Verification items for the finished model (mm, model axes). Face numbers are marked on the shaded views. A direction names the side the tool comes from. Round coordinates to 2 decimals unless told otherwise and drop trailing zeros. Write each loop counter-clockwise with the first axis right and the second up, starting at its lowest first coordinate (ties: lowest second). Pieces come first, ordered by that corner, then holes. Notation, with made-up numbers: (-37, 18) - (21, 18) arc R29 cw to (21, 53) - close; hole circle Ø11 at (-33.5, -27). An arc over 180 degrees is marked (long way). Answer as a JSON object with one key per item and string values.
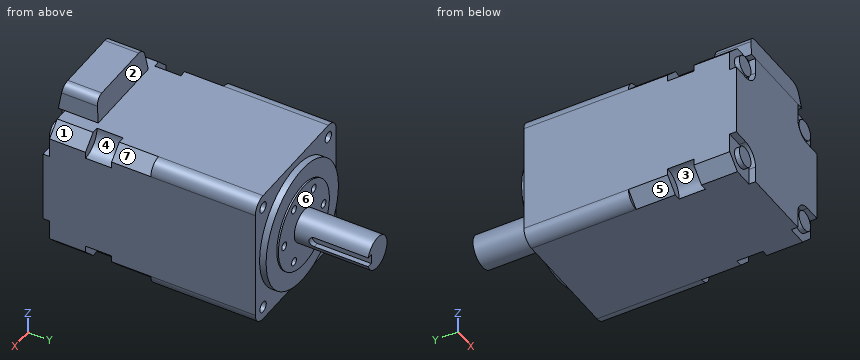
```python
from build123d import *

# Parameters (mm, degrees)
EXTRUDE_1_DEPTH          = 65
CUT_EXTRUDE_1_DEPTH      = 33
CUT_EXTRUDE_START        = -13
CUT_EXTRUDE_2_DEPTH      = 8
CUT_EXTRUDE_3_DEPTH      = 2
SKETCH_5_R               = 3
EXTRUDE_2_DEPTH          = 1.5
SKETCH_6_W               = 26
SKETCH_6_H               = 12.2
EXTRUDE_3_DEPTH          = 7.5
CUT_EXTRUDE_4_REACH      = 80.697
CUT_EXTRUDE_5_REACH      = 76.015
FILLET_2_R               = 2.8
SKETCH_10_R              = 18.8
EXTRUDE_4_DEPTH          = 2
SKETCH_11_R              = 13.25
EXTRUDE_5_DEPTH          = 0.5
SKETCH_12_R              = 5
EXTRUDE_6_DEPTH          = 22.5
CUT_EXTRUDE_6_REACH      = 101.912
CUT_EXTRUDE_6_END_RADIUS = 5
CUT_EXTRUDE_START_2      = 3.2
HOLE_WIZARD_M3_2_D       = 2.5
HOLE_WIZARD_M3_2_DEPTH   = 6.5
HOLE_WIZARD_M3_2_TIP     = 0.751075774
HOLE_WIZARD_M4_1_D       = 3.3
HOLE_WIZARD_M4_1_DEPTH   = 10
HOLE_WIZARD_M4_1_TIP     = 0.991420021


with BuildPart() as part:
    # 草图1 → 凸台-拉伸1 (new body)
    with BuildSketch(Plane(origin=(0, 0, 0), x_dir=(1, 0, 0), z_dir=(0, 1, 0))):
        with BuildLine():
            Line((17, -21), (-17, -21))
            ThreePointArc((-17, -21), (-19.828427125, -19.828427125), (-21, -17))
            Line((-21, -17), (-21, 17))
            ThreePointArc((-21, 17), (-19.828427125, 19.828427125), (-17, 21))
            Line((-17, 21), (17, 21))
            ThreePointArc((17, 21), (19.828427125, 19.828427125), (21, 17))
            Line((21, 17), (21, -17))
            ThreePointArc((21, -17), (19.828427125, -19.828427125), (17, -21))
        make_face()
    extrude(amount=EXTRUDE_1_DEPTH)

    # 草图2 → 切除-拉伸1 (cut)
    with BuildSketch(Plane.XZ):
        with BuildLine():
            Line((-17, 21), (-21, 17))
            ThreePointArc((-21, 17), (-19.828427125, 19.828427125), (-17, 21))
        make_face()
        with BuildLine():
            Line((17, 21), (21, 17))
            ThreePointArc((21, 17), (19.828427125, 19.828427125), (17, 21))
        make_face()
        with BuildLine():
            Line((-21, -17), (-17, -21))
            ThreePointArc((-17, -21), (-19.828427125, -19.828427125), (-21, -17))
        make_face()
        with BuildLine():
            Line((21, -17), (17, -21))
            ThreePointArc((17, -21), (19.828427125, -19.828427125), (21, -17))
        make_face()
    extrude(amount=-CUT_EXTRUDE_1_DEPTH, mode=Mode.SUBTRACT)

    # 草图3 → 切除-拉伸2 (cut)
    with BuildSketch(Plane.XZ.offset(CUT_EXTRUDE_START)):
        with BuildLine():
            Line((-21, 15), (-21, 21))
            Line((-21, 21), (-15, 21))
            ThreePointArc((-15, 21), (-16.757359313, 16.757359313), (-21, 15))
        make_face()
        with BuildLine():
            Line((21, 21), (15, 21))
            ThreePointArc((15, 21), (16.757359313, 16.757359313), (21, 15))
            Line((21, 15), (21, 21))
        make_face()
        with BuildLine():
            Line((-21, -21), (-15, -21))
            ThreePointArc((-15, -21), (-16.757359313, -16.757359313), (-21, -15))
            Line((-21, -15), (-21, -21))
        make_face()
        with BuildLine():
            Line((21, -15), (21, -21))
            Line((21, -21), (15, -21))
            ThreePointArc((15, -21), (16.757359313, -16.757359313), (21, -15))
        make_face()
    extrude(amount=-CUT_EXTRUDE_2_DEPTH, mode=Mode.SUBTRACT)

    # 草图4 → 切除-拉伸3 (cut)
    with BuildSketch(Plane.XZ):
        with BuildLine():
            Line((-21, 21), (-11, 21))
            Line((-11, 21), (-11, 16))
            ThreePointArc((-11, 16), (-12.464466094, 12.464466094), (-16, 11))
            Line((-16, 11), (-21, 11))
            Line((-21, 11), (-21, 21))
        make_face()
        with BuildLine():
            Line((11, 21), (11, 16))
            ThreePointArc((11, 16), (12.464466094, 12.464466094), (16, 11))
            Line((16, 11), (21, 11))
            Line((21, 11), (21, 21))
            Line((21, 21), (11, 21))
        make_face()
        with BuildLine():
            Line((-11, -21), (-11, -16))
            ThreePointArc((-11, -16), (-12.464466094, -12.464466094), (-16, -11))
            Line((-16, -11), (-21, -11))
            Line((-21, -11), (-21, -21))
            Line((-21, -21), (-11, -21))
        make_face()
        with BuildLine():
            Line((21, -21), (11, -21))
            Line((11, -21), (11, -16))
            ThreePointArc((11, -16), (12.464466094, -12.464466094), (16, -11))
            Line((16, -11), (21, -11))
            Line((21, -11), (21, -21))
        make_face()
    extrude(amount=-CUT_EXTRUDE_3_DEPTH, mode=Mode.SUBTRACT)

    # 草图5 → 凸台-拉伸2 (add)
    with BuildSketch(Plane.XZ.offset(-2)):
        with Locations(Location((-15.5, 15.5, 0), (0, 0, 270))):
            Circle(SKETCH_5_R)
        with Locations(Location((15.5, 15.5, 0), (0, 0, 90))):
            Circle(SKETCH_5_R)
        with Locations(Location((15.5, -15.5, 0), (0, 0, 270))):
            Circle(SKETCH_5_R)
        with Locations(Location((-15.5, -15.5, 0), (0, 0, 90))):
            Circle(SKETCH_5_R)
    extrude(amount=EXTRUDE_2_DEPTH)

    # 草图6 → 凸台-拉伸3 (add)
    with BuildSketch(Plane.XY.offset(21)):
        with Locations((0, 6.1)):
            Rectangle(SKETCH_6_W, SKETCH_6_H)
    extrude(amount=EXTRUDE_3_DEPTH)

    # 草图7 → 切除-拉伸4 (cut, up to next)
    with BuildSketch(Plane.ZY.offset(13), mode=Mode.PRIVATE) as cut_extrude_4_sk1:
        Polygon((21, 12.2), (28.5, 11.292400274), (28.5, 12.2), align=None)
    cut_extrude_4_tool1 = extrude(cut_extrude_4_sk1.sketch, amount=-CUT_EXTRUDE_4_REACH, mode=Mode.PRIVATE) & part.part
    # 草图7 → 切除-拉伸4 (cut, up to next)
    with BuildSketch(Plane.ZY.offset(13), mode=Mode.PRIVATE) as cut_extrude_4_sk2:
        Polygon((28.5, 0), (28.5, 0.907599726), (21, 0), align=None)
    cut_extrude_4_tool2 = extrude(cut_extrude_4_sk2.sketch, amount=-CUT_EXTRUDE_4_REACH, mode=Mode.PRIVATE) & part.part
    add(cut_extrude_4_tool1.solids().sort_by_distance((-13, 11.897467, 26))[0], mode=Mode.SUBTRACT)
    add(cut_extrude_4_tool2.solids().sort_by_distance((-13, 0.302533, 26))[0], mode=Mode.SUBTRACT)

    # 草图9 → 切除-拉伸5 (cut, up to next)
    with BuildSketch(Plane.XZ, mode=Mode.PRIVATE) as cut_extrude_5_sk1:
        Polygon((-13, 21), (-12.092400274, 28.5), (-13, 28.5), align=None)
    cut_extrude_5_tool1 = extrude(cut_extrude_5_sk1.sketch, amount=-CUT_EXTRUDE_5_REACH, mode=Mode.PRIVATE) & part.part
    # 草图9 → 切除-拉伸5 (cut, up to next)
    with BuildSketch(Plane.XZ, mode=Mode.PRIVATE) as cut_extrude_5_sk2:
        Polygon((13, 28.5), (13, 21), (12.092400274, 28.5), align=None)
    cut_extrude_5_tool2 = extrude(cut_extrude_5_sk2.sketch, amount=-CUT_EXTRUDE_5_REACH, mode=Mode.PRIVATE) & part.part
    add(cut_extrude_5_tool1.solids().sort_by_distance((-12.697467, 0, 26))[0], mode=Mode.SUBTRACT)
    add(cut_extrude_5_tool2.solids().sort_by_distance((12.697467, 0, 26))[0], mode=Mode.SUBTRACT)

    # 圆角2
    fillet_2_edges = [part.edges().sort_by_distance(p)[0] for p in [
        (-12.092400274, 6.1, 28.5),
        (12.092400274, 6.1, 28.5),
    ]]
    fillet(fillet_2_edges, radius=FILLET_2_R)

    # 草图10 → 凸台-拉伸4 (add)
    with BuildSketch(Plane(origin=(0, 65, 0), x_dir=(1, 0, 0), z_dir=(0, 1, 0))):
        with Locations(Location((0, 0, 0), (0, 0, 270))):
            Circle(SKETCH_10_R)
    extrude(amount=EXTRUDE_4_DEPTH)

    # 草图11 → 凸台-拉伸5 (add)
    with BuildSketch(Plane(origin=(0, 67, 0), x_dir=(1, 0, 0), z_dir=(0, 1, 0))):
        with Locations(Location((0, 0, 0), (0, 0, 270))):
            Circle(SKETCH_11_R)
    extrude(amount=EXTRUDE_5_DEPTH)

    # 草图12 → 凸台-拉伸6 (add)
    with BuildSketch(Plane(origin=(0, 67.5, 0), x_dir=(1, 0, 0), z_dir=(0, 1, 0))):
        with Locations(Location((0, 0, 0), (0, 0, 90))):
            Circle(SKETCH_12_R)
    extrude(amount=EXTRUDE_6_DEPTH)

    # 切除-拉伸6: up to this cylinder (the profile starts inside it)
    cut_extrude_6_end = Plane(origin=(0, 81.75, 0), z_dir=(0, -1, 0)) * Cylinder(CUT_EXTRUDE_6_END_RADIUS, 214.824, mode=Mode.PRIVATE)
    # 草图13 → 切除-拉伸6 (cut, up to the surface)
    with BuildSketch(Plane(origin=(0, 0, 0), x_dir=(0, 0, -1), z_dir=(1, 0, 0)).offset(CUT_EXTRUDE_START_2), mode=Mode.PRIVATE) as cut_extrude_6_sk1:
        with BuildLine():
            Line((1.5, 90), (1.5, 73.5))
            ThreePointArc((1.5, 73.5), (0, 72), (-1.5, 73.5))
            Line((-1.5, 73.5), (-1.5, 90))
            ThreePointArc((-1.5, 90), (0, 91.5), (1.5, 90))
        make_face()
    cut_extrude_6_tool1 = extrude(cut_extrude_6_sk1.sketch, amount=CUT_EXTRUDE_6_REACH, mode=Mode.PRIVATE) & cut_extrude_6_end
    add(cut_extrude_6_tool1.solids().sort_by_distance((3.2, 81.75, 0))[0], mode=Mode.SUBTRACT)

    # M3 螺纹孔2
    with Locations(Plane(origin=(0, 67.5, 0), x_dir=(1, 0, 0), z_dir=(0, 1, 0))):
        with Locations((5.125, 8.876760389), (10.25, 0), (5.125, -8.876760389), (-5.125, -8.876760389), (-10.25, 0), (-5.125, 8.876760389)):
            Hole(HOLE_WIZARD_M3_2_D / 2, depth=HOLE_WIZARD_M3_2_DEPTH)
            with Locations((0, 0, -(HOLE_WIZARD_M3_2_DEPTH + HOLE_WIZARD_M3_2_TIP / 2))):  # 118° drill point
                Cone(0, HOLE_WIZARD_M3_2_D / 2, HOLE_WIZARD_M3_2_TIP, mode=Mode.SUBTRACT)

    # M4 螺纹孔1
    with Locations(Plane(origin=(0, 65, 0), x_dir=(1, 0, 0), z_dir=(0, 1, 0))):
        with Locations((-16.970562748, -16.970562748), (-16.970562748, 16.970562748), (16.970562748, -16.970562748), (16.970562748, 16.970562748)):
            Hole(HOLE_WIZARD_M4_1_D / 2, depth=HOLE_WIZARD_M4_1_DEPTH)
            with Locations((0, 0, -(HOLE_WIZARD_M4_1_DEPTH + HOLE_WIZARD_M4_1_TIP / 2))):  # 118° drill point
                Cone(0, HOLE_WIZARD_M4_1_D / 2, HOLE_WIZARD_M4_1_TIP, mode=Mode.SUBTRACT)


solid = part.part
```
1. Cross-section at D-D (y = 42.5). Record the boundary of the cut face in (x, z), plus the area to 3 significant figures.
Completed:
{"outline": "(-21, -17) arc R4 ccw to (-17, -21) - (17, -21) arc R4 ccw to (21, -17) - (21, 17) arc R4 ccw to (17, 21) - (-17, 21) arc R4 ccw to (-21, 17) - close", "area": "1,750 mm^2"}
2. Cross-section at A-A (y = 16). Record the boundary of the cut face in (x, z).
Completed:
{"outline": "(-21, -15) arc R6 cw to (-15, -21) - (15, -21) arc R6 cw to (21, -15) - (21, 15) arc R6 cw to (15, 21) - (-15, 21) arc R6 cw to (-21, 15) - close"}
3. Cross-section at B-B (x = 0). Record the boundary of the cut face in (y, z).
Completed:
{"outline": "(0, -21) - (65, -21) - (65, -18.8) - (67, -18.8) - (67, -13.25) - (67.5, -13.25) - (67.5, -5) - (90, -5) - (90, 5) - (67.5, 5) - (67.5, 13.25) - (67, 13.25) - (67, 18.8) - (65, 18.8) - (65, 21) - (12.2, 21) - (11.29, 28.5) - (0.91, 28.5) - (0, 21) - close"}
4. Cross-section at C-C (y = 62). Count the separate pieces of the cut face and the enclosed holes in it, plus the area to 3 significant figures.
Completed:
{"separate pieces": "1", "enclosed holes": "10", "area": "1,690 mm^2"}
5. Material ranges on probe 1 along Z at (x, y) = (18, 56); probe 2 along Z at (x, y) = (15.5, 47); probe 3 along Y at (x, z) = (-1.5, 7.5), recorded low to high. Write a range as from..to.
Completed:
{"probe 1": "z = -20.87..-18.26, -15.68..15.68, 18.26..20.87", "probe 2": "z = -21..21", "probe 3": "y = 0..67.5"}
6. Access from +Z, -Z, +X, -X, +Y, -Y to the whole of each face (thin tool, end or side, straight path). Record for the marked faces 5, 6 and 7.
Completed:
{"face 5": "-Z, -X, -Y", "face 6": "+Y", "face 7": "+Z, +X, -Y"}
7. Mould release check, pull along Y, two halves, no side actions. Record for the marked faces 1, 2, 3 and 4: released by +Y, released by -Y, zero draft, split by the parting line, or undercut.
Completed:
{"face 1": "zero draft", "face 2": "released by +Y", "face 3": "undercut", "face 4": "undercut"}
8. Go/stop test with flat-tipped pins: pin 1 (1.8 mm diameter, centred on x = -16, z = -16, fed in from -Y); pin 2 (0.6 mm diameter, centred on y = 1, z = -18.5, fed in from +X); pin 3 (4 mm diameter, centred on y = 74, z = -4.5, fed in from +X). Record where each tip stops, or that it passes through.
Completed:
{"pin 1": "stops at y = 0.5", "pin 2": "stops at x = 16.81", "pin 3": "stops at x = 4.33"}
